from build123d import *

# Parameters (mm, degrees)
F0_W     = 433
F0_H     = 615
F1_DEPTH = 1.5
F2_W     = 1.5
F2_H     = 615
F3_DEPTH = 12.7
F4_R     = 1.5
F6_D     = 6.7564


with BuildPart() as f1:
    # F0 (on Top) → F1 (new body)
    with BuildSketch(Plane.XY):
        Rectangle(F0_W, F0_H)
    extrude(amount=F1_DEPTH)

    # F2 (on face) → F3 (join)
    with BuildSketch(Plane(origin=(0, 0, 0), x_dir=(1, 0, 0), z_dir=(0, 0, -1))):
        with Locations((-215.75, 0)):
            Rectangle(F2_W, F2_H)
        with Locations((215.75, 0)):
            Rectangle(F2_W, F2_H)
    extrude(amount=F3_DEPTH)

    # F4
    f4_edges = [f1.edges().sort_by_distance(p)[0] for p in [
        (-216.5, 0, 1.5),
        (216.5, 0, 1.5),
    ]]
    fillet(f4_edges, radius=F4_R)

    # F6 (through all)
    with Locations(Plane.XY.offset(1.5)):
        with Locations((-118.375, 196.375), (-51.7, 196.375), (14.975, 196.375), (81.65, 196.375), (148.325, 196.375), (148.325, -143.35), (81.65, -143.35), (14.975, -143.35), (-51.7, -143.35), (-118.375, -143.35), (-185.05, 196.375), (-185.05, -143.35)):
            Hole(F6_D / 2)


solid = f1.part
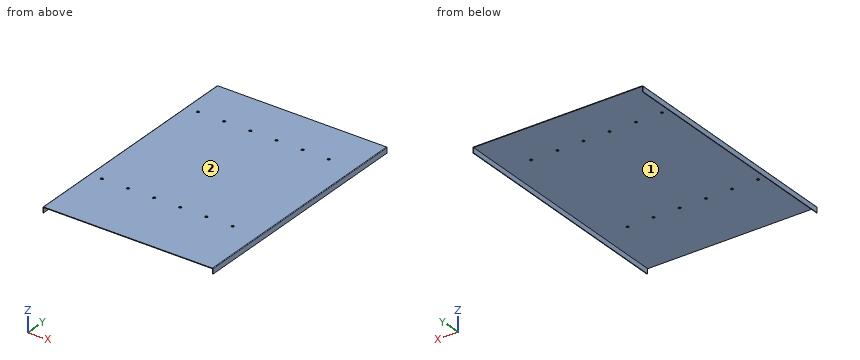
The listing builds one solid part. Answer for the finished solid, in the listing's coordinates (mm). Face numbers are marked on the shaded views. Round coordinates to 2 decimals unless told otherwise and drop trailing zeros. Loops run counter-clockwise (first coordinate to the right, second up) from the corner with the lowest first, then second, coordinate; pieces in that order, holes last. Notation, with made-up numbers: M 1.5,43 L 36.5,43 A20 ccw 36.5,47 Z; hole C -4.5,43.5 d1. An arc over 180 degrees is marked long. Return JSON: item names as keys, results as strings.
Q1. The mould has two halves that part along X. Classify the marked faces 1 and 2: released by +X, released by -X, zero draft, split by the parting line, or undercut.
Results list:
{"face 1": "undercut", "face 2": "zero draft"}
Q2. Find the intervals of material crossed by line 1 along Y through (x, z) = (-51.7, 0.45); line 2 along X through (y, z) = (224, -2.75); line 3 along Z through (x, y) = (-122, -150), in increasing order. Write a range as from..to.
Results list:
{"line 1": "y = -307.5..-146.73, -139.97..193, 199.75..307.5", "line 2": "x = -216.5..-215, 215..216.5", "line 3": "z = 0..1.5"}
Q3. Find section A-A, the plane z = -10.25. Determine the outline of the cut face in (x, y).
Results list:
{"outline": "M -216.5,-307.5 L -215,-307.5 L -215,307.5 L -216.5,307.5 Z; M 215,-307.5 L 216.5,-307.5 L 216.5,307.5 L 215,307.5 Z"}
Q4. Find section C-C, the plane x = 180. Determine the outline of the cut face in (y, z), plus the area to 4 significant figures.
Results list:
{"outline": "M -307.5,0 L 307.5,0 L 307.5,1.5 L -307.5,1.5 Z", "area": "922.5 mm2"}
Q5. Find section B-B, the plane y = 224. Determine the outline of the cut face in (x, z).
Results list:
{"outline": "M -216.5,-12.7 L -215,-12.7 L -215,0 L 215,0 L 215,-12.7 L 216.5,-12.7 L 216.5,0 A1.5 ccw 215,1.5 L -215,1.5 A1.5 ccw -216.5,0 Z"}
Q6. This flat-tipped pin is pushed along its axis until it touches: pin 1 Ø11 at (x, y) = (81.65, 196.375) entering from -Z. Where does it stop, or does it pass through?
Results list:
{"pin 1": "stops at z = 0"}
